Check sheet for the modelled part. Datum: model origin and axes. Units: mm. A direction names the side the tool comes from. Round coordinates to 2 decimals unless told otherwise and drop trailing zeros. Write each loop counter-clockwise with the first axis right and the second up, starting at its lowest first coordinate (ties: lowest second). Pieces come first, ordered by that corner, then holes.
Item 1: Section check A-A, the plane x = 0. Record the cut outline in (y, z).
Item 2: Release check for a two-part mould opening along Z. For faces 1 (the flat face through (-33, 26, -200)), 2 (the cylindrical face through (16.33, 16.94, 28.1)), 3 (the flat face through (26, 30, -100)) record: pulls with the +Z half, pulls with the -Z half, needs draft (parallel to the pull), parting line crosses it, or undercut.
Item 3: Material ranges on line 1 along X through (y, z) = (9.75, 0); line 2 along Z through (x, y) = (0, 22.5); line 3 along Z through (x, y) = (11, 12.5), recorded low to high.
Item 4: Section check C-C, the plane z = -72. Record the cut outline in (x, y), plus the area to 3 significant figures.
Item 5: Section check D-D, the plane y = 25.5. State how many separate pieces and enclosed holes the cut face has, plus the area to 3 significant figures.
Item 6: Section check B-B, the plane y = 2.5. Record the cut outline in (x, z) (3 decimals).
Item 7: Set-up check for faces 4 (the flat face through (11.27, 25.56, 30.96)), 5 (the flat face through (-11.27, 25.56, 30.96)), 6 (the flat face through (-22, 16, -101)), 7 (the flat face through (-26, 26, -42.936)): record each of +Z, -Z, +X, -X, +Y, -Y from which the full face is reachable in a straight line by a thin tool's end or side.
Item 8: Depth check by flat-ended pin: pin 1 (4 mm diameter, centred on x = -14, z = -24.25, fed in from -Y); pin 2 (11 mm diameter, centred on x = -21, z = -221, fed in from +Y); pin 3 (9 mm diameter, centred on x = -24.5, y = 27, fed in from +Z). Enter the tip coordinate at first touch or a pass-through.
Autodesk Inventor part; units mm, degrees
ref_plane "YZ Plane" through (0, 0, 0) normal (1, 0, 0) x (0, 1, 0)
ref_plane "XZ Plane" through (0, 0, 0) normal (0, 1, 0) x (-1, 0, 0)
ref_plane "XY Plane" through (0, 0, 0) normal (0, 0, 1) x (1, 0, 0)
sketch "Boceto1" plane through (0, 0, 0) normal (0, 1, 0) x (-1, 0, 0)
  circle A0 centre (0, 0) radius 37
  circle A1 centre (0, -200) radius 37
  line L0 (0, 0) -> (0, -200)
  line L1 (30, -21.6564) -> (30, -178.3436)
  line L2 (-30, -21.6564) -> (-30, -178.3436)
  line L3 (36.4379, -6.425) -> (30, -42.9361)
  line L4 (0, -100) -> (14.5981, -100)
  line L5 (36.4379, -193.575) -> (30, -157.0639)
  line L6 (-36.4379, -6.425) -> (-30, -42.9361)
  line L7 (-36.4379, -193.575) -> (-30, -157.0639)
  point P0 (-36.4379, -6.425)
  point P1 (-30, -42.9361)
  point P2 (-30, -157.0639)
  point P3 (-36.4379, -193.575)
  dimension "d0" = 200
  dimension "d1" = 74
  dimension "d2" = 74
  dimension "d3" = 60
  dimension "d4" = 170
extrude "Extrusión1" add sketch "Boceto1" along normal blind 30
sketch "Boceto2" plane through (0, 0, 0) normal (0, -1, 0) x (1, 0, 0)
  circle A0 centre (0, 0) radius 37.1
  dimension "d7" = 74.2
extrude "Extrusión2" cut sketch "Boceto2" against normal blind 7
sketch "Boceto3" plane through (0, 30, 0) normal (0, 1, 0) x (1, 0, 0)
  circle A0 centre (0, 0) radius 43.1
  arc A1 (36.4379, 193.575) -> (-36.4379, 193.575) centre (0, 200) ccw
  circle A2 centre (0, 200) radius 29
  line L0 (-28.5594, 194.9642) -> (-22, 157.7639)
  line L1 (-36.4379, 193.575) -> (-30, 157.0639)
  line L2 (-22, 157.7639) -> (-22, 42.2361)
  line L3 (-30, 157.0639) -> (-30, 42.9361)
  line L4 (0, 0) -> (0, 200)
  line L5 (28.5594, 194.9642) -> (22, 157.7639)
  line L6 (22, 157.7639) -> (22, 42.2361)
  circle A3 centre (0, 0) radius 29
  line L7 (-22, 42.2361) -> (-28.5594, 5.0358)
  line L8 (22, 42.2361) -> (28.5594, 5.0358)
  line L9 (-30, 42.9361) -> (-36.4379, 6.425)
  line L10 (36.4379, 6.425) -> (30, 42.9361)
  point P0 (-22, 37.0622)
  point P1 (22, 37.0622)
  point P2 (22, 37.0622)
  point P3 (28.5594, 194.9642)
  point P4 (-23.0228, 36.4357)
  point P5 (23.0228, 36.4357)
  dimension "d10" = 86.2
  dimension "d11" = 58
  dimension "d12" = 8
  dimension "d60" = 58
extrude "Extrusión3" cut sketch "Boceto3" against normal blind 24 contours A0 L4 A2 L5 L6 L8 | L7 L2 L0 A2 L4 A0 | A2
sketch "Boceto5" plane through (0, 30, 0) normal (0, 1, 0) x (1, 0, 0)
  circle A0 centre (0, 0) radius 29
  circle A1 centre (0, 0) radius 43.1
  line L0 (-23.0228, 36.4357) -> (-28.5594, 5.0358)
  line L1 (23.0228, 36.4357) -> (28.5594, 5.0358)
  line L2 (-30, 42.9361) -> (-36.4379, 6.425)
  line L3 (36.4379, 6.425) -> (30, 42.9361)
  dimension "d15" = 58
  dimension "d16" = 86.2
extrude "Extrusión4" cut sketch "Boceto5" against normal blind 17 contours A0 | A0 L0 A1 L1 picked at (2.6828, 38.1473)
sketch "Boceto6" plane through (0, 13, 0) normal (0, 1, 0) x (1, 0, 0)
  circle A0 centre (0, 0) radius 28
  circle A1 centre (14, -24.2487) radius 1.7
  circle A2 centre (28, 0) radius 1.7
  circle A3 centre (14, 24.2487) radius 1.7
  circle A4 centre (-14, 24.2487) radius 1.7
  circle A5 centre (-28, 0) radius 1.7
  circle A6 centre (-14, -24.2487) radius 1.7
  line L0 (-0.7827, -11.2442) -> (-0.7827, 11.3946)
  line L1 (0, 0) -> (-14, -24.2487)
  dimension "d19" = 56
  dimension "d20" = 3.4
  dimension "d23" = 360
  dimension "d34" = 30
extrude "Extrusión5" cut sketch "Boceto6" along normal through all both and the other way through all contours A0 A2 | A0 A2 | A3 A0 | A0 A3 | A1 A0 | A0 A1 | A4 A0 | A0 A4 | A6 A0 | A0 L1 A6 | A0 A6 L1 | A5 A0 | A0 A5
sketch "Boceto7" plane through (0, 13, 0) normal (0, 1, 0) x (1, 0, 0)
  circle A0 centre (-14, -24.2487) radius 1.7
  circle A1 centre (-14, -24.2487) radius 4.5
  circle A2 centre (14, -24.2487) radius 4.5
  circle A3 centre (28, 0) radius 4.5
  circle A4 centre (14, 24.2487) radius 4.5
  circle A5 centre (-14, 24.2487) radius 4.5
  circle A6 centre (-28, 0) radius 4.5
  point P0 (0, 0)
  dimension "d27" = 9
  dimension "d30" = 360
extrude "Extrusión6" cut sketch "Boceto7" along normal through all contours A0 | A1 | A2 | A3 | A4 | A5 | A6
sketch "Boceto8" plane through (0, 13, 0) normal (0, 1, 0) x (1, 0, 0)
  circle A0 centre (0, 0) radius 15
  dimension "d35" = 30
extrude "Extrusión7" cut sketch "Boceto8" against normal through all
sketch "Boceto9" plane through (0, 30, 0) normal (0, 1, 0) x (1, 0, 0)
  arc A0 (28.5594, 194.9642) -> (-28.5594, 194.9642) centre (0, 200) ccw
  circle A1 centre (0, 200) radius 29
  circle A2 centre (0, 200) radius 37
  line L0 (0, 200) -> (-18.5, 232.0429)
  line L1 (0, 200) -> (0, 0)
  line L2 (0, 0) -> (-12.6547, -34.7686)
  arc A3 (-36.4379, 6.425) -> (36.4379, 6.425) centre (0, 0) ccw
  line L3 (0, 0) -> (-35.7393, -9.5763)
  line L4 (-30, 42.9361) -> (-22, 42.9361)
  line L5 (-22, 42.9361) -> (-22, 82.9361)
  line L6 (-22, 82.9361) -> (-30, 82.9361)
  line L7 (-30, 42.9361) -> (-30, 82.9361)
  line L8 (-30, 157.0639) -> (-22, 157.0639)
  line L9 (-22, 117.0639) -> (-30, 117.0639)
  line L10 (-30, 157.0639) -> (-30, 117.0639)
  line L11 (0, 200) -> (-37, 200)
  line L12 (-22, 117.0639) -> (-22, 157.0639)
  line L13 (-22, 42.2361) -> (-22, 157.7639)
  line L14 (0, 200) -> (18.5, 232.0429)
  line L15 (0, 0) -> (12.6547, -34.7686)
  line L16 (0, 0) -> (35.7393, -9.5763)
  line L17 (30, 42.9361) -> (22, 42.9361)
  line L18 (22, 42.9361) -> (22, 82.9361)
  line L19 (22, 82.9361) -> (30, 82.9361)
  line L20 (30, 42.9361) -> (30, 82.9361)
  line L21 (30, 157.0639) -> (22, 157.0639)
  line L22 (22, 117.0639) -> (30, 117.0639)
  line L23 (30, 157.0639) -> (30, 117.0639)
  line L24 (0, 200) -> (37, 200)
  line L25 (22, 117.0639) -> (22, 157.0639)
  circle A4 centre (0, 0) radius 29
  circle A5 centre (0, 0) radius 37
  point P0 (-22, 37.0622)
  point P1 (22, 37.0622)
  point P2 (22, 157.7639)
  point P3 (14.5, 225.1147)
  point P4 (29, 200)
  point P5 (-29, 200)
  point P6 (-14.5, 225.1147)
  point P7 (28.0118, -7.5058)
  point P8 (9.9186, -27.2511)
  point P9 (35.7393, -9.5763)
  point P10 (-9.9186, -27.2511)
  point P11 (-28.0118, -7.5058)
  dimension "d38" = 30
  dimension "d39" = 20
  dimension "d40" = 55
  dimension "d41" = 40
  dimension "d42" = 40
extrude "Extrusión8" cut sketch "Boceto9" against normal blind 9 contours A0 L14 A2 L24 | A0 L11 A2 L0 | A4 L2 A3 L3 | A4 L16 A3 L15 | L7 L6 L5 L4 | L9 L10 L8 L12 | L17 L18 L19 L20 | L23 L22 L25 L21
sketch "Boceto10" plane through (0, 21, 0) normal (0, 1, 0) x (1, 0, 0)
  circle A0 centre (-26, 62.9361) radius 2.05
  circle A1 centre (-26, 137.0639) radius 2.05
  arc A2 (-29, 200) -> (-28.5594, 194.9642) centre (0, 200) ccw
  circle A3 centre (0, 200) radius 33
  circle A4 centre (-28.5788, 216.5) radius 2.05
  circle A5 centre (0, 0) radius 33
  circle A6 centre (-28.5788, -16.5) radius 2.05
  line L0 (-30, 42.9361) -> (-30, 82.9361)
  line L1 (-30, 82.9361) -> (-22, 82.9361)
  line L2 (-30, 117.0639) -> (-30, 157.0639)
  line L3 (-22, 117.0639) -> (-30, 117.0639)
  line L4 (0, 200) -> (-28.5788, 216.5)
  line L5 (0, 0) -> (-28.5788, -16.5)
  line L6 (0, 0) -> (0, 200)
  circle A7 centre (26, 62.9361) radius 2.05
  circle A8 centre (26, 137.0639) radius 2.05
  circle A9 centre (28.5788, 216.5) radius 2.05
  circle A10 centre (28.5788, -16.5) radius 2.05
  line L7 (0, 200) -> (28.5788, 216.5)
  line L8 (0, 0) -> (28.5788, -16.5)
  dimension "d45" = 66
  dimension "d46" = 66
  dimension "d47" = 4.1
  dimension "d48" = 4
  dimension "d49" = 20
  dimension "d50" = 4
  dimension "d51" = 20
  dimension "d53" = 60
  dimension "d54" = 60
extrude "Extrusión9" cut sketch "Boceto10" against normal blind 5.8 contours A0 | A1 | A9 L7 A3 | A3 A9 | L7 A9 A3 | A4 A3 | A3 L4 A4 | A3 A4 L4 | A6 L5 A5 | A5 A6 | A10 A5 | A5 L8 A10 | L5 A6 A5 | L8 A5 A10 | A7 | A8
sketch "Boceto11" plane through (0, 6, 0) normal (0, 1, 0) x (1, 0, 0)
  arc A0 (14.5, 225.1147) -> (-14.5, 225.1147) centre (0, 200) ccw
  circle A1 centre (0, 200) radius 9
  point P0 (0, 0)
  dimension "d57" = 18
extrude "Extrusión10" cut sketch "Boceto11" against normal through all
sketch "Boceto12" plane through (0, 13, 0) normal (0, 1, 0) x (1, 0, 0)
  circle A0 centre (0, 42) radius 7
  point P0 (0, 0)
  dimension "d61" = 14
  dimension "d62" = 42
extrude "Extrusión11" cut sketch "Boceto12" against normal blind 4
chamfer "Chaflán1" distance 0.7 angle 45 1 edges at (-9, 6, -200)
equation "\"d5\" = altura"
equation "\"altura\" = 30"
properties part number "Tercer segmento - superior" material "Plastico PETG"
Values found:
1. outline: (0, -237) - (30, -237) - (30, -229) - (6, -229) - (6, -209.7) - (5.3, -209) - (0, -209) - close; (0, -191) - (5.3, -191) - (6, -190.3) - (6, -43.1) - (9, -43.1) - (9, -35) - (13, -35) - (13, -15) - (7, -15) - (7, -37.1) - (0, -37.1) - close; (7, 15) - (13, 15) - (13, 29) - (30, 29) - (30, 37) - (7, 37) - close
2. face 1: pulls with the -Z half
2. face 2: undercut
2. face 3: needs draft
3. line 1: x = -37 to -29.7, -26.3 to -15, 15 to 26.3, 29.7 to 37
3. line 2: z = -237 to -229, 29 to 37
3. line 3: z = -235.33 to -226.83, -41.67 to -10.2, 10.2 to 35.33
4. outline: (-30, 0) - (30, 0) - (30, 21) - (22, 21) - (22, 6) - (-22, 6) - (-22, 21) - (-30, 21) - close
4. area: 600 mm2
5. separate pieces: 8
5. enclosed holes: 0
5. area: 2,490 mm2
6. outline: (-36.438, -193.575) arc R37 ccw (long way) to (36.438, -193.575) - (30, -157.064) - (30, -42.936) - (35.965, -9.106) arc R37.1 cw to (-35.965, -9.106) - (-30, -42.936) - (-30, -157.064) - close; hole circle Ø18 at (0, -200)
7. face 4: +X, +Y
7. face 5: -X, +Y
7. face 6: +Y
7. face 7: +X, -X, +Y
8. pin 1: stops at y = 7
8. pin 2: stops at y = 21
8. pin 3: stops at z = 7.77
